from build123d import *

# Parameters (mm, degrees)
F0_W     = 26.815738529
F0_H     = 56.2547557056
F1_DEPTH = 25.4
F2_W     = 18.9459016547
F2_H     = 11.3675417379
F3_DEPTH = 12.5
F4_W     = 1.2322755065
F4_H     = 1.9270461053
F5_DEPTH = 1
F6_R     = 0.1393490387
F7_DEPTH = 60


# Not quite as in the source:
# - a feature names something its author has since deleted; it is built from what else it names


with BuildPart() as f1:
    # F0 (on Front) → F1 (new body)
    with BuildSketch(Plane.XZ):
        Rectangle(F0_W, F0_H)
    extrude(amount=F1_DEPTH)

    # F2 (on face) → F3 (cut, symmetric)
    with BuildSketch(Plane(origin=(0, 0, -28.1273778528), x_dir=(1, 0, 0), z_dir=(0, 0, -1))):
        with Locations((0.7286877371, 11.9504923932)):
            Rectangle(F2_W, F2_H)
    extrude(amount=F3_DEPTH, both=True, mode=Mode.SUBTRACT)

    # F4 (on face) → F5 (join)
    with BuildSketch(Plane.XY.offset(28.1273778528)):
        with Locations((0, -11.4252325147)):
            Rectangle(F4_W, F4_H)
    extrude(amount=F5_DEPTH)

    # F6 (on face) → F7 (join)
    with BuildSketch(Plane.XY.offset(29.1273778528)):
        with Locations((0, -11.4126661792)):
            Circle(F6_R)
    extrude(amount=F7_DEPTH)


solid = f1.part
Input: part model. Units: mm. Frame: model coordinates. A direction names the side the tool comes from. Give positions to 0.01 mm unless a question says otherwise; leave off trailing zeros. Write each loop counter-clockwise with the first axis right and the second up, starting at its lowest first coordinate (ties: lowest second). Pieces come first, ordered by that corner, then holes.
Q1. Section A-A, the plane z = -20.5. Output: boundary loops of the cut face in (x, y), plus the area to 3 significant figures.
Q2. Material intervals for probe 1 along X at (y, z) = (-8.25, -22); probe 2 along Z at (x, y) = (-3.25, -23.75); probe 3 along Z at (x, y) = (2, -14.5), sorted ascending.
Q3. Section C-C, the plane x = -4. Output: boundary loops of the cut face in (y, z), plus the area to 3 significant figures.
Q4. Set-up query: faces 1 (the face through (-13.408, -13, 0)), 2 (the face through (1, -12, -15.627)). Return all of +Z, -Z, +X, -X, +Y, -Y with unobstructed straight access to the full face (end or side cutting, diameter ignored); none if empty.
Q5. First-contact query: P1, Ø9, axis at x = -0.5, y = -11, coming from the -Z side; P2, Ø0.5, axis at x = 0, z = 28.5, coming from the -Y side; P3, Ø1.5, axis at x = -5.5, y = -12.5, coming from the +Z side. Flat tips, straight axial feed; report the tip coordinate or a pass-through.
Q6. Pull-direction query (Y, two-part tool) for faces 3 (the face through (0, 0, 0)), 4 (the face through (10.202, -12, -22)), 5 (the face through (0, -13, 28.127)); classes: pulls with the +Y half, pulls with the -Y half, needs draft (parallel to the pull), parting line crosses it, or undercut.
Q7. Section D-D, the plane z = 54. Output: boundary loops of the cut face in (x, y).
Q8. Section B-B, the plane y = -8.5. Output: boundary loops of the cut face in (x, z).
Filled in:
1. outline: (-13.41, -25.4) - (13.41, -25.4) - (13.41, 0) - (-13.41, 0) - close; hole (-8.74, -17.63) - (10.2, -17.63) - (10.2, -6.27) - (-8.74, -6.27) - close
1. area: 466 mm2
2. probe 1: x = -13.41 to -8.74, 10.2 to 13.41
2. probe 2: z = -28.13 to 28.13
2. probe 3: z = -15.63 to 28.13
3. outline: (-25.4, -28.13) - (-17.63, -28.13) - (-17.63, -15.63) - (-6.27, -15.63) - (-6.27, -28.13) - (0, -28.13) - (0, 28.13) - (-25.4, 28.13) - close
3. area: 1,290 mm2
4. face 1: +Z, -Z, -X, +Y, -Y
4. face 2: -Z
5. P1: stops at z = -15.63
5. P2: stops at y = -12.39
5. P3: stops at z = 28.13
6. face 3: pulls with the +Y half
6. face 4: undercut
6. face 5: needs draft
7. outline: circle Ø0.28 at (0, -11.41)
8. outline: (-13.41, -28.13) - (-8.74, -28.13) - (-8.74, -15.63) - (10.2, -15.63) - (10.2, -28.13) - (13.41, -28.13) - (13.41, 28.13) - (-13.41, 28.13) - close
